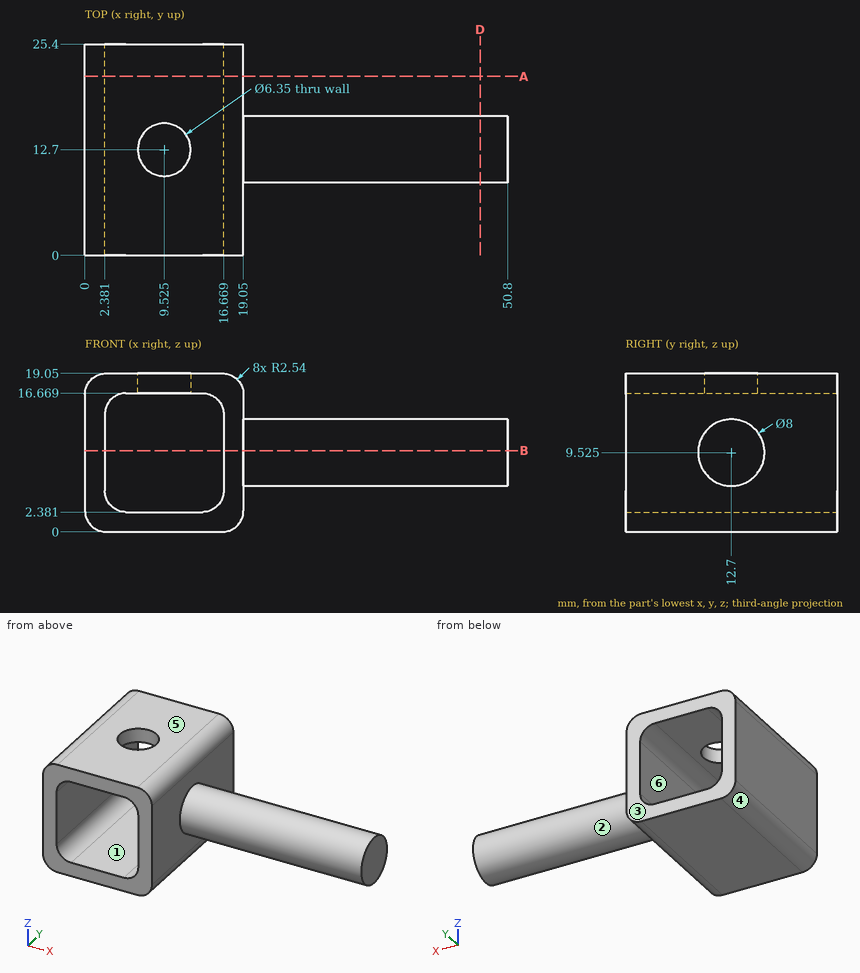
Geometry check sheet. Reference: drawing and pictorial views, mm from the part's lowest x, y, z. A direction names the side the tool comes from. Give positions to 0.01 mm unless a question says otherwise; leave off trailing zeros. Loops run counter-clockwise (first coordinate to the right, second up) from the corner with the lowest first, then second, coordinate; pieces in that order, holes last. Notation, with made-up numbers: (54.5, 34) - (75.5, 34) arc R24 ccw to (75.5, 71) - close; hole circle Ø2 at (13, 60.25). An arc over 180 degrees is marked (long way). One line per question, with ' | ' between items. Start each with the question number.
1. Cross-section at D-D, the plane x = 47.5. Enter the section's corners in (y, z) (1 decimal).
2. Draft check along X on the marked faces 4, 5 and 6. Enter one of: released by +X, released by -X, zero draft, split by the parting line, or undercut.
3. Gauge pin test, flat ends, axial feed: pin 1 Ø1.5 at (x, z) = (41.5, 11.5) entering from +Y; pin 2 Ø3 at (x, z) = (26.5, 7.5) entering from +Y; pin 3 Ø1 at (x, y) = (18.5, 13.5) entering from -Z. Record the tip position at first contact, or that the pin passes through.
4. Cross-section at B-B, the plane z = 9.75. Enter the section's corners in (x, y).
5. Cross-section at A-A, the plane y = 21.5. Enter the section's corners in (x, z), plus the area to 3 significant figures.
6. Material ranges on line 1 along X through (y, z) = (14.75, 12); line 2 along Z through (x, y) = (8, 8.5), recorded low to high. Write a range as [from, to].
7. Set-up check for the marked faces 1, 2 and 3: record each of +Z, -Z, +X, -X, +Y, -Y from which the full face is reachable in a straight line by a thin tool's end or side.
Check result:
1) outline: circle Ø8 at (12.7, 9.5)
2) face 4: released by -X | face 5: zero draft | face 6: undercut
3) pin 1: stops at y = 16.51 | pin 2: stops at y = 16.67 | pin 3: stops at z = 0.48
4) outline: (0, 0) - (2.38, 0) - (2.38, 25.4) - (0, 25.4) - close; (16.67, 0) - (19.05, 0) - (19.05, 8.71) - (50.8, 8.71) - (50.8, 16.69) - (19.05, 16.69) - (19.05, 25.4) - (16.67, 25.4) - close
5) outline: (0, 2.54) arc R2.54 ccw to (2.54, 0) - (16.51, 0) arc R2.54 ccw to (19.05, 2.54) - (19.05, 16.51) arc R2.54 ccw to (16.51, 19.05) - (2.54, 19.05) arc R2.54 ccw to (0, 16.51) - close; hole (2.38, 4.92) arc R2.54 ccw to (4.92, 2.38) - (14.13, 2.38) arc R2.54 ccw to (16.67, 4.92) - (16.67, 14.13) arc R2.54 ccw to (14.13, 16.67) - (4.92, 16.67) arc R2.54 ccw to (2.38, 14.13) - close | area: 159 mm2
6) line 1: x = [0, 2.38], [16.67, 50.8] | line 2: z = [0, 2.38], [16.67, 19.05]
7) face 1: +Y, -Y | face 2: +X | face 3: +Z, -Z, +X, -X, +Y
